Model file for the job. Use its own axes, mm. A direction names the side the tool comes from. Coordinates: 2 decimals unless noted, no trailing zeros. Order: outer loops, then holes, each group sorted by start corner. A loop starts at its lowest first (then second) coordinate and runs counter-clockwise, first axis right, second up. Notation, with made-up numbers: (74, 40) -> (96, 40) arc R30 ccw to (96, 79) -> close; hole circle Ø11 at (-21.5, 3). An arc over 180 degrees is marked (long way). Write item = value, one per line. Start each with the question number.
Q1. 3-axis set-ups, long thin cutter, end or side, ignore diameter. For faces 5 (the face through (22, 0, 8)), 6 (the face through (47.147, 8.217, 7.888)): which of +Z, -Z, +X, -X, +Y, -Y reach the whole face in a straight line?
Q2. Flat gauge pins, fed straight in: pin 1 (1.5 mm diameter, centred on y = 4, z = 9.5, fed in from -X); pin 2 (2 mm diameter, centred on y = 1, z = 4, fed in from +X); pin 3 (1 mm diameter, centred on x = 28, y = 7.5, fed in from +Z); pin 4 (8.5 mm diameter, centred on x = 8, z = 8, fed in from -Y). Where does each tip first touch, or does it go through?
Q3. Mould opens along Z. For faces 1 (the face through (22, 9.5, 8)), 2 (the face through (5.236, 9.254, 10.534)), 3 (the face through (5.236, -0.246, 10.534)), 4 (the face through (0.002, 9.246, 8.176)) say: +Z half, -Z half, draft (parallel to the pull), parting line (faces both ways), or undercut.
Q4. Cut at C-C, the plane x = 10.5. List the corners of the cut face in (y, z).
Q5. Wall check: line 1 (Z direction, x = 8, y = -0.4); line 2 (Y direction, x = 43, z = 8); line 3 (Y direction, x = 45, z = 2.75). Give the ranges that are in metal, low to high. Write a range as from..to.
Q6. Cut at D-D, the plane z = 2. List the corners of the cut face in (x, y).
Q7. Cut at B-B, the plane z = 9.5. List the corners of the cut face in (x, y).
Q8. Cut at A-A, the plane x = 30.5. List the corners of the cut face in (y, z).
from build123d import *

# Parameters (mm, degrees)
BASE_FLANGE1_DEPTH  = 16
CUT_EXTRUDE1_DEPTH  = 53.04084934
SKETCH7_R           = 3.75
BOSS_EXTRUDE1_DEPTH = 2
CUT_EXTRUDE2_START  = -2
SKETCH8_R           = 3.75
CUT_EXTRUDE2_DEPTH  = 2
BOSS_EXTRUDE2_START = -2
SKETCH9_R           = 3.75
BOSS_EXTRUDE2_DEPTH = 2
CUT_EXTRUDE4_START  = -2
SKETCH10_R          = 3.75
CUT_EXTRUDE4_DEPTH  = 2


# Sheet-metal steps are written as plain solids
with BuildPart() as part:
    # Sketch1 → Base-Flange1 (new body)
    with BuildSketch(Plane.XY):
        with BuildLine():
            Line((0, 0), (44, 0))
            ThreePointArc((44, 0), (46.828427125, 1.171572875), (48, 4))
            Line((48, 4), (48, 5))
            ThreePointArc((48, 5), (46.828427125, 7.828427125), (44, 9))
            Line((44, 9), (0, 9))
            Line((0, 9), (0, 9.5))
            Line((0, 9.5), (44, 9.5))
            ThreePointArc((44, 9.5), (47.181980515, 8.181980515), (48.5, 5))
            Line((48.5, 5), (48.5, 4))
            ThreePointArc((48.5, 4), (47.181980515, 0.818019485), (44, -0.5))
            Line((44, -0.5), (0, -0.5))
            Line((0, -0.5), (0, 0))
        make_face()
    extrude(amount=BASE_FLANGE1_DEPTH)

    # Sketch6 → Cut-Extrude1 (cut, through all)
    with BuildSketch(Plane.XZ.offset(0.5)):
        with BuildLine():
            Line((8, 0), (8, -3.97427409))
            Line((8, -3.97427409), (-3.94829055, -3.97427409))
            Line((-3.94829055, -3.97427409), (-3.94829055, 19.074328647))
            Line((-3.94829055, 19.074328647), (8, 19.074328647))
            Line((8, 19.074328647), (8, 16))
            ThreePointArc((8, 16), (0, 8), (8, 0))
        make_face()
    extrude(amount=-CUT_EXTRUDE1_DEPTH, mode=Mode.SUBTRACT)

    # Sketch7 → Boss-Extrude1 (add)
    with BuildSketch(Plane(origin=(0, 9.5, 0), x_dir=(1, 0, 0), z_dir=(0, 1, 0))):
        with Locations(Location((8, -8, 0), (0, 0, 180))):
            Circle(SKETCH7_R)
    extrude(amount=-BOSS_EXTRUDE1_DEPTH)

    # Sketch8 → Cut-Extrude2 (cut)
    with BuildSketch(Plane.XZ.offset(-7.5).offset(CUT_EXTRUDE2_START)):
        with Locations((8, 8)):
            Circle(SKETCH8_R)
    extrude(amount=CUT_EXTRUDE2_DEPTH, mode=Mode.SUBTRACT)

    # Sketch9 → Boss-Extrude2 (add)
    with BuildSketch(Plane.XZ.offset(0.5).offset(BOSS_EXTRUDE2_START)):
        with Locations((8, 8)):
            Circle(SKETCH9_R)
    extrude(amount=BOSS_EXTRUDE2_DEPTH)

    # Sketch10 → Cut-Extrude4 (cut)
    with BuildSketch(Plane.XZ.offset(0.5).offset(CUT_EXTRUDE4_START)):
        with Locations((8, 8)):
            Circle(SKETCH10_R)
    extrude(amount=CUT_EXTRUDE4_DEPTH, mode=Mode.SUBTRACT)


solid = part.part
Here are the results:
q1.face_5 = +Z, -Z, -X
q1.face_6 = +Z, -Z, +X, +Y
q2.pin_1 = 47.93
q2.pin_2 = 48.03
q2.pin_3 = through
q2.pin_4 = -0.5
q3.face_1 = draft
q3.face_2 = undercut
q3.face_3 = undercut
q3.face_4 = parting line
q4.outline = (-0.5, 0) -> (0, 0) -> (0, 5.2) -> (-0.5, 5.2) -> close; (-0.5, 10.8) -> (0, 10.8) -> (0, 16) -> (-0.5, 16) -> close; (9, 0) -> (9.5, 0) -> (9.5, 5.2) -> (9, 5.2) -> close; (9, 10.8) -> (9.5, 10.8) -> (9.5, 16) -> (9, 16) -> close
q5.line_1 = 0..4.25, 11.75..16
q5.line_2 = -0.5..0, 9..9.5
q5.line_3 = -0.39..0.13, 8.87..9.39
q6.outline = (2.71, -0.5) -> (44, -0.5) arc R4.5 ccw to (48.5, 4) -> (48.5, 5) arc R4.5 ccw to (44, 9.5) -> (2.71, 9.5) -> (2.71, 9) -> (44, 9) arc R4 cw to (48, 5) -> (48, 4) arc R4 cw to (44, 0) -> (2.71, 0) -> close
q7.outline = (0.14, -0.5) -> (4.56, -0.5) -> (4.56, 0) -> (0.14, 0) -> close; (0.14, 9) -> (4.56, 9) -> (4.56, 9.5) -> (0.14, 9.5) -> close; (11.44, -0.5) -> (44, -0.5) arc R4.5 ccw to (48.5, 4) -> (48.5, 5) arc R4.5 ccw to (44, 9.5) -> (11.44, 9.5) -> (11.44, 9) -> (44, 9) arc R4 cw to (48, 5) -> (48, 4) arc R4 cw to (44, 0) -> (11.44, 0) -> close
q8.outline = (-0.5, 0) -> (0, 0) -> (0, 16) -> (-0.5, 16) -> close; (9, 0) -> (9.5, 0) -> (9.5, 16) -> (9, 16) -> close
